The model under review builds one solid part; all positions refer to its coordinate system, in mm. Face numbers are marked on the shaded views. A direction names the side the tool comes from. Round coordinates to 2 decimals unless told otherwise and drop trailing zeros. Order: outer loops, then holes, each group sorted by start corner. A loop starts at its lowest first (then second) coordinate and runs counter-clockwise, first axis right, second up. Notation, with made-up numbers: M 77,43.25 L 134,43.25 A27 ccw 134,76.25 Z; hole C -30,86.5 d2. An arc over 180 degrees is marked long. Answer as a JSON object with one key per item and string values. Group by question number.
1) Consider section B-B, the plane z = 55. Count the separate pieces of the cut face and the enclosed holes in it, then the cut area to 3 significant figures.
2) Consider section A-A, the plane y = 78. Write out the cut boundary in (x, z) (3 decimals).
3) Insertion check: pin 1 Ø6 at (x, z) = (-236, 15) entering from +Y; pin 2 Ø1 at (x, z) = (242, 95.5) entering from -Y; pin 3 Ø0.5 at (y, z) = (174, 59.5) entering from +X (3 decimals). Each pin has a flat end and moves straight along its axis. Give the tip position at first contact, or say it passes through.
4) For the marked faces 1, 2 and 3, list the 3-axis set-ups (+Z, -Z, +X, -X, +Y, -Y) from which the entire face can be reached by the end or side of a thin tool; tool diameter is ignored.
5) To check wall thickness, follow line 1 (Z direction, x = -140, y = 191.5) (3 decimals). State the ranges of the line that lie inside material, in increasing order.
```python
from build123d import *

# Parameters (mm, degrees)
F0_W     = 1.5875
F0_H     = 107.95
F1_DEPTH = 314.325
F2_W     = 655.1622450352
F2_H     = 386.0229451675
F3_DEPTH = 3.175


with BuildPart() as f1:
    # F0 (on Right) → F1 (new body, symmetric)
    with BuildSketch(Plane.YZ):
        with Locations((348.45625, 53.975)):
            Rectangle(F0_W, F0_H)
    extrude(amount=F1_DEPTH, both=True)



with BuildPart() as f1b:
    # F0 (on Right) → F1, piece 2 (new body, symmetric)
    with BuildSketch(Plane.YZ):
        with Locations((313.53125, 53.975)):
            Rectangle(F0_W, F0_H)
    extrude(amount=F1_DEPTH, both=True)


with BuildPart() as f1c:
    # F0 (on Right) → F1, piece 3 (new body, symmetric)
    with BuildSketch(Plane.YZ):
        with Locations((278.60625, 53.975)):
            Rectangle(F0_W, F0_H)
    extrude(amount=F1_DEPTH, both=True)


with BuildPart() as f1d:
    # F0 (on Right) → F1, piece 4 (new body, symmetric)
    with BuildSketch(Plane.YZ):
        with Locations((243.68125, 53.975)):
            Rectangle(F0_W, F0_H)
    extrude(amount=F1_DEPTH, both=True)


with BuildPart() as f1e:
    # F0 (on Right) → F1, piece 5 (new body, symmetric)
    with BuildSketch(Plane.YZ):
        with Locations((208.75625, 53.975)):
            Rectangle(F0_W, F0_H)
    extrude(amount=F1_DEPTH, both=True)


with BuildPart() as f1f:
    # F0 (on Right) → F1, piece 6 (new body, symmetric)
    with BuildSketch(Plane.YZ):
        with Locations((173.83125, 53.975)):
            Rectangle(F0_W, F0_H)
    extrude(amount=F1_DEPTH, both=True)


with BuildPart() as f1g:
    # F0 (on Right) → F1, piece 7 (new body, symmetric)
    with BuildSketch(Plane.YZ):
        with Locations((138.90625, 53.975)):
            Rectangle(F0_W, F0_H)
    extrude(amount=F1_DEPTH, both=True)


with BuildPart() as f1h:
    # F0 (on Right) → F1, piece 8 (new body, symmetric)
    with BuildSketch(Plane.YZ):
        with Locations((103.98125, 53.975)):
            Rectangle(F0_W, F0_H)
    extrude(amount=F1_DEPTH, both=True)


with BuildPart() as f1i:
    # F0 (on Right) → F1, piece 9 (new body, symmetric)
    with BuildSketch(Plane.YZ):
        with Locations((69.05625, 53.975)):
            Rectangle(F0_W, F0_H)
    extrude(amount=F1_DEPTH, both=True)


with BuildPart() as f1j:
    # F0 (on Right) → F1, piece 10 (new body, symmetric)
    with BuildSketch(Plane.YZ):
        with Locations((34.13125, 53.975)):
            Rectangle(F0_W, F0_H)
    extrude(amount=F1_DEPTH, both=True)


with BuildPart() as f1k:
    # F0 (on Right) → F1, piece 11 (new body, symmetric)
    with BuildSketch(Plane.YZ):
        with Locations((-0.79375, 53.975)):
            Rectangle(F0_W, F0_H)
    extrude(amount=F1_DEPTH, both=True)


with BuildPart() as f1_1:
    add(f1.part)

    add(f1b.part)  # F3 merges F1b

    add(f1c.part)  # F3 merges F1c

    add(f1d.part)  # F3 merges F1d

    add(f1e.part)  # F3 merges F1e

    add(f1f.part)  # F3 merges F1f

    add(f1g.part)  # F3 merges F1g

    add(f1h.part)  # F3 merges F1h

    add(f1i.part)  # F3 merges F1i

    add(f1j.part)  # F3 merges F1j

    add(f1k.part)  # F3 merges F1k
    # F2 (on Top) → F3 (join)
    with BuildSketch(Plane.XY):
        with Locations((12.5250071287, 190.857162117)):
            Rectangle(F2_W, F2_H)
    extrude(amount=F3_DEPTH)


solid = f1_1.part
```
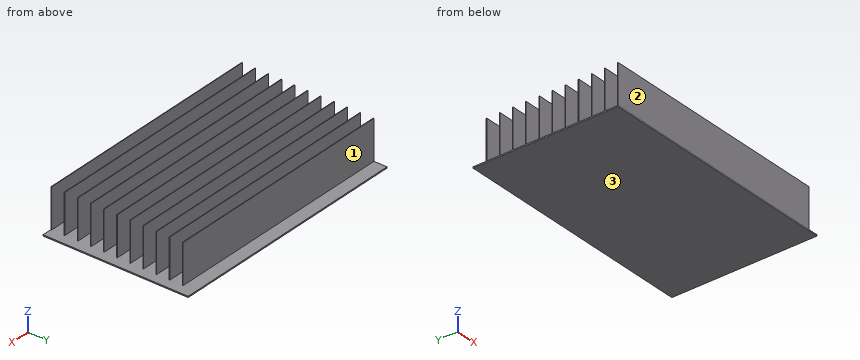
Results list:
{
 "1": {"separate pieces": "11", "enclosed holes": "0", "area": "11,000 mm^2"},
 "2": {"outline": "M -315.056,0 L 340.106,0 L 340.106,3.175 L -315.056,3.175 Z"},
 "3": {"pin 1": "y = 349.25", "pin 2": "y = -1.59", "pin 3": "x = 314.325"},
 "4": {"face 1": "+Z, +X, -X, +Y", "face 2": "+Z, +X, -X, -Y", "face 3": "-Z, +X, -X, +Y, -Y"},
 "5": {"line 1": "0 to 3.175"}
}
